from build123d import *

# Parameters (mm, degrees)
ESQUISSE1_W        = 50.2
ESQUISSE1_H        = 28.2
BOSS_EXTRU_1_DEPTH = 1.6
D_GAGEMENT_M31_D   = 3.4
CONG_1_R           = 3
ESQUISSE5_R        = 3.691889044
ESQUISSE5_W        = 6.611446916
ESQUISSE5_H        = 9.58403545
ESQUISSE5_W_2      = 4.100122118
ESQUISSE5_H_2      = 7.636477445
ESQUISSE5_W_3      = 9.789041557
ESQUISSE5_H_3      = 9.789041557
BOSS_EXTRU_2_DEPTH = 10.4


with BuildPart() as part:
    # Esquisse1 → Boss.-Extru.1 (new body)
    with BuildSketch(Plane.XY):
        Rectangle(ESQUISSE1_W, ESQUISSE1_H)
    extrude(amount=BOSS_EXTRU_1_DEPTH)

    # Dégagement M31 (through all)
    with Locations(Plane.XY.offset(1.6)):
        with Locations((-21.5, 10.5), (21.5, 10.5), (21.5, -10.5), (-21.5, -10.5)):
            Hole(D_GAGEMENT_M31_D / 2)

    # Congé1
    cong_1_edges = [part.edges().sort_by_distance(p)[0] for p in [
        (-25.1, 14.1, 0.8),
        (25.1, 14.1, 0.8),
        (25.1, -14.1, 0.8),
        (-25.1, -14.1, 0.8),
    ]]
    fillet(cong_1_edges, radius=CONG_1_R)

    # Esquisse5 → Boss.-Extru.2 (add)
    with BuildSketch(Plane.XY.offset(1.6)):
        with Locations((-10.301556822, 9.481532398)):
            Circle(ESQUISSE5_R)
        with Locations(Location((10.301556822, 9.481532398, 0), (0, 0, 180))):
            Circle(ESQUISSE5_R)
        with Locations((-20.884997039, 0)):
            Rectangle(ESQUISSE5_W, ESQUISSE5_H)
        with Locations((20.884997039, 0)):
            Rectangle(ESQUISSE5_W, ESQUISSE5_H)
        with Locations((-2.511324797, 8.635882212)):
            Rectangle(ESQUISSE5_W_2, ESQUISSE5_H_2)
        with Locations((10.480937165, -7.303342522)):
            Rectangle(ESQUISSE5_W_3, ESQUISSE5_H_3)
    extrude(amount=BOSS_EXTRU_2_DEPTH)


solid = part.part
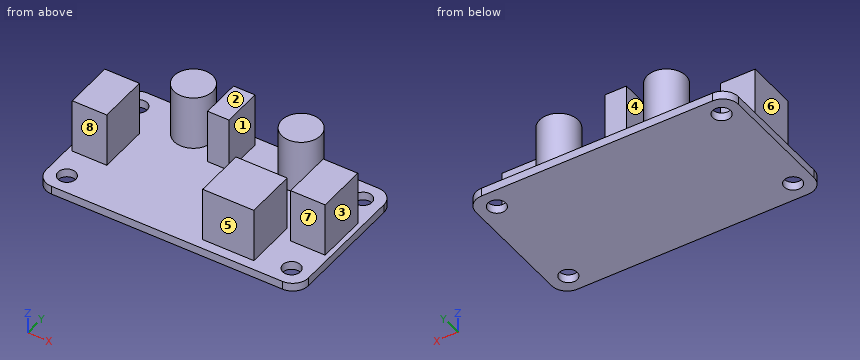
Geometry: final body of the model. Coordinates: model frame, mm. Face numbers are marked on the shaded views. A direction names the side the tool comes from. Give positions to 0.01 mm unless a question says otherwise; leave off trailing zeros. Write each loop counter-clockwise with the first axis right and the second up, starting at its lowest first coordinate (ties: lowest second). Pieces come first, ordered by that corner, then holes.
(1) Cut plane C-C, the plane z = 1. Return loops of the section in (x, y).
(2) Cut plane D-D, the plane y = -7. Return loops of the section in (x, z), then the cut area to 3 significant figures.
(3) Cut plane A-A, the plane x = -21.5. Return loops of the section in (y, z), then the cut area to 3 significant figures.
(4) Cut plane B-B, the plane y = -10.5. Return loops of the section in (x, z).
(5) Mould query, pull axis X, two halves, no side actions, for the marked faces 1, 2, 3 and 4. Classes: released by +X, released by -X, zero draft, split by the parting line, or undercut.
(6) First-contact query: P1, Ø4.5, axis at x = -21.5, y = -10.5, coming from the +Z side; P2, Ø2, axis at x = -21, z = 7, coming from the +Y side; P3, Ø5, axis at y = 0.5, z = 7, coming from the -X side. Flat tips, straight axial feed; report the tip coordinate or a pass-through.
(7) Access query for the marked faces 5, 6, 7 and 8. Directions: +Z, -Z, +X, -X, +Y, -Y. A direction counts if a zero-diameter tool reaches every point of the face in a straight line with its end or side. Return the directions, or none.
(8) Ray query, line 1 (Y direction, x = -21.5, z = 0.3); line 2 (X direction, y = -4.5, z = 11.25); line 3 (X direction, y = 2.25, z = 3.5). Return the intervals inside material, ascending.
Values follow:
1. outline: (-25.1, -11.1) arc R3 ccw to (-22.1, -14.1) - (22.1, -14.1) arc R3 ccw to (25.1, -11.1) - (25.1, 11.1) arc R3 ccw to (22.1, 14.1) - (-22.1, 14.1) arc R3 ccw to (-25.1, 11.1) - close; hole circle Ø3.4 at (-21.5, -10.5); hole circle Ø3.4 at (-21.5, 10.5); hole circle Ø3.4 at (21.5, -10.5); hole circle Ø3.4 at (21.5, 10.5)
2. outline: (-25.1, 0) - (25.1, 0) - (25.1, 1.6) - (15.38, 1.6) - (15.38, 12) - (5.59, 12) - (5.59, 1.6) - (-25.1, 1.6) - close
2. area: 182 mm2
3. outline: (-14.1, 0) - (-12.2, 0) - (-12.2, 1.6) - (-14.1, 1.6) - close; (-8.8, 0) - (8.8, 0) - (8.8, 1.6) - (4.79, 1.6) - (4.79, 12) - (-4.79, 12) - (-4.79, 1.6) - (-8.8, 1.6) - close; (12.2, 0) - (14.1, 0) - (14.1, 1.6) - (12.2, 1.6) - close
3. area: 134 mm2
4. outline: (-25.1, 0) - (-23.2, 0) - (-23.2, 1.6) - (-25.1, 1.6) - close; (-19.8, 0) - (19.8, 0) - (19.8, 1.6) - (15.38, 1.6) - (15.38, 12) - (5.59, 12) - (5.59, 1.6) - (-19.8, 1.6) - close; (23.2, 0) - (25.1, 0) - (25.1, 1.6) - (23.2, 1.6) - close
5. face 1: undercut
5. face 2: zero draft
5. face 3: released by +X
5. face 4: undercut
6. P1: stops at z = 1.6
6. P2: stops at y = 4.79
6. P3: stops at x = -24.19
7. face 5: +Z, +X, -X, -Y
7. face 6: +Z, -X, +Y, -Y
7. face 7: +Z, +X, -Y
7. face 8: +Z, -X, -Y
8. line 1: y = -14.1 to -12.2, -8.8 to 8.8, 12.2 to 14.1
8. line 2: x = -24.19 to -17.58, 5.59 to 15.38, 17.58 to 24.19
8. line 3: x = -24.19 to -17.58, 17.58 to 24.19
